Work out the finished part from the listing and answer in its coordinate system (mm). Face numbers are marked on the shaded views. A direction names the side the tool comes from. Give positions to 0.01 mm unless a question says otherwise; leave off trailing zeros. Loops run counter-clockwise (first coordinate to the right, second up) from the corner with the lowest first, then second, coordinate; pieces in that order, holes last. Notation, with made-up numbers: (75.25, 68) -> (83.25, 68) arc R23 cw to (83.25, 82) -> close; hole circle Ø3 at (-34.75, 68). An arc over 180 degrees is marked (long way). Answer as CSV lines item,"result". Start each with the question number.
1. Find section D-D, the plane y = 5.5. Give the vertices of the cut face in (x, z).
2. A tool of negligible diameter and unlimited length cuts with its end or side. For the marked faces 1, 2 and 3, from which of +Z, -Z, +X, -X, +Y, -Y can it reach the whole face along a straight path? Write none if from no direction.
3. Determine the mould class of the marked faces 4, 5, 6 and 7 for opening direction X: +X half, -X half, draft (parallel to the pull), parting line (faces both ways), or undercut.
4. Find the intervals of material crossed by line 1 along Y through (x, z) = (27.5, 17.5); line 2 along X through (y, z) = (-35, 17); line 3 along Y through (x, z) = (82, 19), in increasing order.
5. Find section C-C, the plane z = 4.25. Give the vertices of the cut face in (x, y), and give its area (3 significant figures).
6. Find section B-B, the plane y = 32.5. Give the vertices of the cut face in (x, z), and give its area (3 significant figures).
7. Find section A-A, the plane x = 30. Give the vertices of the cut face in (y, z), and give its area (3 significant figures).
8. A flat-ended cylindrical pin translates along its axis: pin 1 Ø12 at (x, y) = (62, -24) entering from -Z. Find the tip coordinate at first contact, or state that the pin passes through.
Autodesk Inventor part; units mm, degrees
ref_plane "YZ Plane" through (0, 0, 0) normal (1, 0, 0) x (0, 1, 0)
ref_plane "XZ Plane" through (0, 0, 0) normal (0, 1, 0) x (-1, 0, 0)
ref_plane "XY Plane" through (0, 0, 0) normal (0, 0, 1) x (1, 0, 0)
sketch "Sketch1" plane through (0, 0, 0) normal (0, 0, 1) x (1, 0, 0)
  point P0 (0, 0)
sketch "LAYER1" plane through (0, 0, 0) normal (0, 0, 1) x (1, 0, 0)
  line L0 (70, 20.5) -> (90, 20.5)
  line L1 (90, 20.5) -> (90, 57.5)
  line L2 (90, 57.5) -> (0, 57.5)
  line L3 (0, 57.5) -> (0, -57.5)
  line L4 (0, -57.5) -> (90, -57.5)
  line L5 (90, -57.5) -> (90, -20.5)
  line L6 (90, -20.5) -> (70, -20.5)
  line L7 (70, -20.5) -> (70, -37.5)
  line L8 (70, -37.5) -> (20, -37.5)
  line L9 (20, -37.5) -> (20, 37.5)
  line L10 (20, 37.5) -> (70, 37.5)
  line L11 (70, 37.5) -> (70, 20.5)
sketch "LAYER2" plane through (0, 0, 0) normal (0, 0, 1) x (1, 0, 0)
  line L0 (20.1, -20) -> (110.1, -20)
  line L1 (110.1, -20) -> (110.1, 20)
  line L2 (110.1, 20) -> (20.1, 20)
  line L3 (20.1, 20) -> (20.1, -20)
sketch "LAYER3" plane through (0, 0, 0) normal (0, 0, 1) x (1, 0, 0)
  line L0 (20.5, -71.2) -> (69.5, -71.2)
  line L1 (69.5, -71.2) -> (69.5, -58)
  line L2 (69.5, -58) -> (20.5, -58)
  line L3 (20.5, -58) -> (20.5, -71.2)
sketch "LAYER4" plane through (0, 0, 0) normal (0, 0, 1) x (1, 0, 0)
  line L0 (20.5, -23.8) -> (69.5, -23.8)
  line L1 (69.5, -23.8) -> (69.5, -37)
  line L2 (69.5, -37) -> (20.5, -37)
  line L3 (20.5, -37) -> (20.5, -23.8)
sketch "LAYER5" plane through (0, 0, 0) normal (0, 0, 1) x (1, 0, 0)
  line L0 (20.5, 23.8) -> (69.5, 23.8)
  line L1 (69.5, 23.8) -> (69.5, 37)
  line L2 (69.5, 37) -> (20.5, 37)
  line L3 (20.5, 37) -> (20.5, 23.8)
sketch "LAYER6" plane through (0, 0, 0) normal (0, 0, 1) x (1, 0, 0)
  line L0 (20.5, 71.2) -> (69.5, 71.2)
  line L1 (69.5, 71.2) -> (69.5, 58)
  line L2 (69.5, 58) -> (20.5, 58)
  line L3 (20.5, 58) -> (20.5, 71.2)
extrude "Extrusion1" add sketch "LAYER1" along normal blind 20
properties part number "Core"
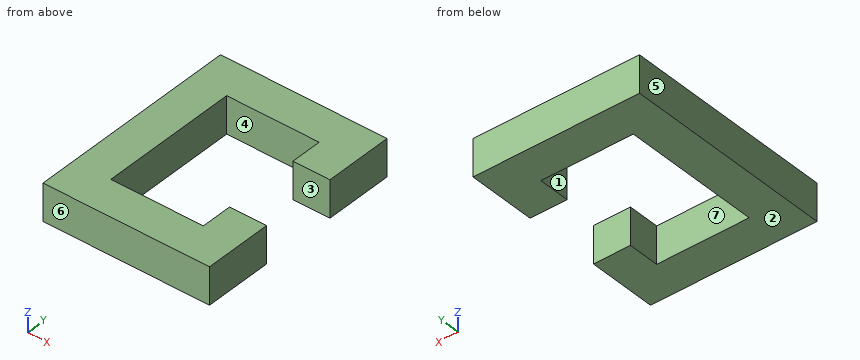
Resolved:
1,outline,"(0, 0) -> (20, 0) -> (20, 20) -> (0, 20) -> close"
2,face 1,"+Z, -Z"
2,face 2,"-Z, +X, -X, +Y, -Y"
2,face 3,"+Z, -Z, +X"
3,face 4,"undercut"
3,face 5,"-X half"
3,face 6,"draft"
3,face 7,"undercut"
4,line 1,"y = -57.5 to -37.5, 37.5 to 57.5"
4,line 2,"x = 0 to 20, 70 to 90"
4,line 3,"y = -57.5 to -20.5, 20.5 to 57.5"
5,outline,"(0, -57.5) -> (90, -57.5) -> (90, -20.5) -> (70, -20.5) -> (70, -37.5) -> (20, -37.5) -> (20, 37.5) -> (70, 37.5) -> (70, 20.5) -> (90, 20.5) -> (90, 57.5) -> (0, 57.5) -> close"
5,area,"5,780 mm^2"
6,outline,"(0, 0) -> (20, 0) -> (20, 20) -> (0, 20) -> close; (70, 0) -> (90, 0) -> (90, 20) -> (70, 20) -> close"
6,area,"800 mm^2"
7,outline,"(-57.5, 0) -> (-37.5, 0) -> (-37.5, 20) -> (-57.5, 20) -> close; (37.5, 0) -> (57.5, 0) -> (57.5, 20) -> (37.5, 20) -> close"
7,area,"800 mm^2"
8,pin 1,"passes through"
